```python
from build123d import *

# Parameters (mm, degrees)
SKETCH1_W           = 43
SKETCH1_H           = 43
BOSS_EXTRUDE1_DEPTH = 48
CHAMFER1_SIZE       = 2.5
SKETCH2_R           = 11
BOSS_EXTRUDE2_DEPTH = 2
SKETCH3_R           = 2.5
BOSS_EXTRUDE3_DEPTH = 20
SKETCH4_R           = 1.5
CUT_EXTRUDE1_DEPTH  = 10


with BuildPart() as part:
    # Sketch1 → Boss-Extrude1 (new body)
    with BuildSketch(Plane.XY):
        Rectangle(SKETCH1_W, SKETCH1_H)
    extrude(amount=BOSS_EXTRUDE1_DEPTH)

    # Chamfer1
    chamfer1_edges = [part.edges().sort_by_distance(p)[0] for p in [
        (21.5, -21.5, 24),
        (-21.5, -21.5, 24),
        (-21.5, 21.5, 24),
        (21.5, 21.5, 24),
    ]]
    chamfer(chamfer1_edges, length=CHAMFER1_SIZE)

    # Sketch2 → Boss-Extrude2 (add)
    with BuildSketch(Plane.XY.offset(48)):
        Circle(SKETCH2_R)
    extrude(amount=BOSS_EXTRUDE2_DEPTH)

    # Sketch3 → Boss-Extrude3 (add)
    with BuildSketch(Plane.XY.offset(50)):
        Circle(SKETCH3_R)
    extrude(amount=BOSS_EXTRUDE3_DEPTH)

    # Sketch4 → Cut-Extrude1 (cut)
    with BuildSketch(Plane.XY.offset(48)):
        with Locations((-15.5, 15.5)):
            Circle(SKETCH4_R)
        with Locations((15.5, 15.5)):
            Circle(SKETCH4_R)
        with Locations((15.5, -15.5)):
            Circle(SKETCH4_R)
        with Locations((-15.5, -15.5)):
            Circle(SKETCH4_R)
    extrude(amount=-CUT_EXTRUDE1_DEPTH, mode=Mode.SUBTRACT)


solid = part.part
```
The model under review builds one solid part; all positions refer to its coordinate system, in mm. A direction names the side the tool comes from. Give positions to 0.01 mm unless a question says otherwise; leave off trailing zeros. Loops run counter-clockwise (first coordinate to the right, second up) from the corner with the lowest first, then second, coordinate; pieces in that order, holes last. Notation, with made-up numbers: (77.25, -12) - (131.25, -12) arc R27 cw to (131.25, 12) - close; hole circle Ø2 at (-14, 35.5). An arc over 180 degrees is marked (long way). Answer as a JSON object with one key per item and string values.
Q1. Mouldability with a two-part tool opening along X and no side actions: class faces 3 (the flat face through (-16, 16, 38)), 4 (the cylindrical face through (-0.54, -2.44, 59.86)), 5 (the flat face through (0, 0, 0)), 6 (the flat face through (20.3, -20.2, 23.7)) as +X half, -X half, draft (parallel to the pull), parting line (faces both ways), or undercut.
Worked out:
{"face 3": "undercut", "face 4": "parting line", "face 5": "draft", "face 6": "+X half"}
Q2. To check wall thickness, follow line 1 along Y through (x, z) = (-15.5, 42); line 2 along Y through (x, z) = (-15, 45); line 3 along Z through (x, y) = (-19, -2). State the ranges of each line that lie inside material, in increasing order.
Worked out:
{"line 1": "y = -21.5 to -17, -14 to 14, 17 to 21.5", "line 2": "y = -21.5 to -16.91, -14.09 to 14.09, 16.91 to 21.5", "line 3": "z = 0 to 48"}
Q3. For faces 1 (the cylindrical face through (14, 15.57, 43.07)), 2 (the flat face through (20.2, 20.3, 23.7)), list the 3-axis set-ups (+Z, -Z, +X, -X, +Y, -Y) from which the entire face can be reached by the end or side of a thin tool; tool diameter is ignored.
Worked out:
{"face 1": "+Z", "face 2": "+Z, -Z, +X, +Y"}
Q4. Add section C-C on z = 40. State the section outline as (x, y) points, plus the area to 3 significant figures.
Worked out:
{"outline": "(-21.5, -19) - (-19, -21.5) - (19, -21.5) - (21.5, -19) - (21.5, 19) - (19, 21.5) - (-19, 21.5) - (-21.5, 19) - close; hole circle Ø3 at (-15.5, -15.5); hole circle Ø3 at (-15.5, 15.5); hole circle Ø3 at (15.5, -15.5); hole circle Ø3 at (15.5, 15.5)", "area": "1,810 mm^2"}
Q5. Add section D-D on z = 62. State the section outline as (x, y) points.
Worked out:
{"outline": "circle Ø5 at (0, 0)"}
Q6. Add section B-B on y = 0. State the section outline as (x, z) points.
Worked out:
{"outline": "(-21.5, 0) - (21.5, 0) - (21.5, 48) - (11, 48) - (11, 50) - (2.5, 50) - (2.5, 70) - (-2.5, 70) - (-2.5, 50) - (-11, 50) - (-11, 48) - (-21.5, 48) - close"}
Q7. Insertion check: pin 1 (2.5 mm diameter, centred on x = 16, y = 16, fed in from +Z); pin 2 (2.5 mm diameter, centred on x = 15.5, y = 15.5, fed in from +Z); pin 3 (12 mm diameter, centred on x = -11.5, y = 7, fed in from +Z). Each pin has a flat end and moves straight along its axis. Give the tip position at first contact, or say it passes through.
Worked out:
{"pin 1": "stops at z = 48", "pin 2": "stops at z = 38", "pin 3": "stops at z = 50"}
Q8. Add section A-A on x = -15.5. State the section outline as (y, z) points, plus the area to 3 significant figures.
Worked out:
{"outline": "(-21.5, 0) - (21.5, 0) - (21.5, 48) - (17, 48) - (17, 38) - (14, 38) - (14, 48) - (-14, 48) - (-14, 38) - (-17, 38) - (-17, 48) - (-21.5, 48) - close", "area": "2,000 mm^2"}
